Source: CAD feature listing. Evaluate the final solid. Frame: model axes, mm. A direction names the side the tool comes from. Round coordinates to 2 decimals unless told otherwise and drop trailing zeros. Order: outer loops, then holes, each group sorted by start corner. A loop starts at its lowest first (then second) coordinate and runs counter-clockwise, first axis right, second up. Notation, with made-up numbers: M 72,-23.75 L 113,-23.75 A14 ccw 113,-12.75 Z; hole C 84.25,69 d5. An arc over 180 degrees is marked long. Use CSV: the item, a comma, the result in double quotes. Start each with the question number.
```python
from build123d import *

# Parameters (mm, degrees)
SKETCH1_R           = 1.47
BOSS_EXTRUDE1_DEPTH = 1.5875


with BuildPart() as part:
    # Sketch1 → Boss-Extrude1 (new body, symmetric)
    with BuildSketch(Plane.XY):
        Polygon((-12.5, 35), (-35, 35), (-35, 12.5), (-38.175, 12.5), (-38.175, -12.5), (-35, -12.5), (-35, -35), (-12.5, -35), (-12.5, -31.825), (-1.47, -31.825), (-1.47, -28.125), (-3.25, -28.125), (-3.25, -25.525), (-1.47, -25.525), (-1.47, -21.825), (1.47, -21.825), (1.47, -25.525), (3.25, -25.525), (3.25, -28.125), (1.47, -28.125), (1.47, -31.825), (12.5, -31.825), (12.5, -35), (35, -35), (35, -12.5), (38.175, -12.5), (38.175, 12.5), (35, 12.5), (35, 35), (12.5, 35), (12.5, 31.825), (1.47, 31.825), (1.47, 28.125), (3.25, 28.125), (3.25, 25.525), (1.47, 25.525), (1.47, 21.825), (-1.47, 21.825), (-1.47, 25.525), (-3.25, 25.525), (-3.25, 28.125), (-1.47, 28.125), (-1.47, 31.825), (-12.5, 31.825), align=None)
        with Locations((-36.5875, 0)):
            Circle(SKETCH1_R, mode=Mode.SUBTRACT)
        with Locations((36.5875, 0)):
            Circle(SKETCH1_R, mode=Mode.SUBTRACT)
    extrude(amount=BOSS_EXTRUDE1_DEPTH, both=True)


solid = part.part
```
(1) Draft query along X for faces 4 (the face through (24, 35, 0)), 5 (the face through (-35, 24, 0)), 6 (the face through (35, 24, 0)), 7 (the face through (-37.754, -0.894, -0.022)). Return one class per face: pulls with the +X half, pulls with the -X half, needs draft (parallel to the pull), parting line crosses it, or undercut.
(2) Line query: line 1 along Y through (x, z) = (-2.5, 0.6) (3 decimals); line 2 along X through (y, z) = (14, 1.15); line 3 along Y through (x, z) = (-9.5, 0) (3 decimals). Output: solid intervals per line, ascending.
(3) Contact query for flat-ended pins moving along their axis: P1, Ø1.6, axis at y = 31, z = 0, coming from the -X side; P2, Ø1.4, axis at x = -2.5, z = -0.5, coming from the -Y side (3 decimals); P3, Ø1.6, axis at y = 29, z = 0.5, coming from the +X side; P4, Ø4.5, axis at x = -36.59, y = 0, coming from the -Z side. Output: stop coordinate, or through.
(4) Section A-A on y = 0. Give the number of separate pieces and of enclosed holes in the cut face, plus the area to 3 significant figures.
(5) Reachability of faces 1 (the face through (1.47, 24, 0)), 2 (the face through (-35, -24, 0)), 3 (the face through (-2, -28.125, 0)) from +Z, -Z, +X, -X, +Y, -Y: full face, straight path, thin tool, end or side. Return the list, or none.
(6) Section C-C on y = -15. Return loops of the section in (x, z), plus the area to 3 significant figures.
(7) Section D-D on x = -8. Return loops of the section in (y, z) (1 decimal).
Results below:
1,face 4,"needs draft"
1,face 5,"pulls with the -X half"
1,face 6,"pulls with the +X half"
1,face 7,"undercut"
2,line 1,"y = -31.825 to -28.125, -25.525 to 25.525, 28.125 to 31.825"
2,line 2,"x = -35 to 35"
2,line 3,"y = -31.825 to 31.825"
3,P1,"stops at x = -35"
3,P2,"stops at y = -31.825"
3,P3,"stops at x = 35"
3,P4,"stops at z = -1.59"
4,separate pieces,"3"
4,enclosed holes,"0"
4,area,"224 mm2"
5,face 1,"+Z, -Z, +Y"
5,face 2,"+Z, -Z, -X, -Y"
5,face 3,"+Z, -Z"
6,outline,"M -35,-1.59 L 35,-1.59 L 35,1.59 L -35,1.59 Z"
6,area,"222 mm2"
7,outline,"M -31.8,-1.6 L 31.8,-1.6 L 31.8,1.6 L -31.8,1.6 Z"
